The figure shows three views and two pictorial views of one solid part (mm, origin at its lowest corner). Answer the questions. A direction names the side the tool comes from. Coordinates: 2 decimals unless noted, no trailing zeros. Loops run counter-clockwise (first coordinate to the right, second up) from the corner with the lowest first, then second, coordinate; pieces in that order, holes last. Notation, with made-up numbers: M 38.5,-23 L 87.5,-23 A14 ccw 87.5,-6 Z; hole C 65.25,-21 d2. An arc over 180 degrees is marked long. Return JSON: item names as keys, results as strings. Group by question number.
1. Given P1, Ø3, axis at x = 20.5, z = 108.5, coming from the -Y side; P2, Ø2, axis at y = 323.5, z = 159.5, coming from the -X side; P3, Ø3, axis at x = 5.5, y = 253.5, coming from the +Z side; P4, Ø6, axis at x = 21, z = 110, coming from the +Y side, each flat-ended and moving along its own axis, determine where each tip first touches the part or whether it passes through.
2. The mould has two halves that part along Y. Classify the marked faces 1, 2, 3 and 4: pulls with the +Y half, pulls with the -Y half, needs draft (parallel to the pull), parting line crosses it, or undercut.
3. Straight lines are drawn through the part: L1, parallel to Z at x = 8.5, y = 28.5; L2, parallel to Z at x = 1.5, y = 92.5; L3, parallel to Y at x = 19.75, z = 166. For each, find the intervals that lie inside material, in ascending order. Write a range as from..to.
4. Section C-C (y = 89.5) is taken. Write down the section's boundary in (x, z), then the cut area to 3 significant figures.
5. Which of the six approach directions +Z, -Z, +X, -X, +Y, -Y give full straight-line access (tool end or side, diameter ignored) to the marked faces 5, 6 and 7?
6. Section B-B (z = 73.5) is taken. Write down the section's boundary in (x, y).
7. Section A-A (x = 18.75) is taken. Write down the section's boundary in (y, z), then the cut area to 3 significant figures.
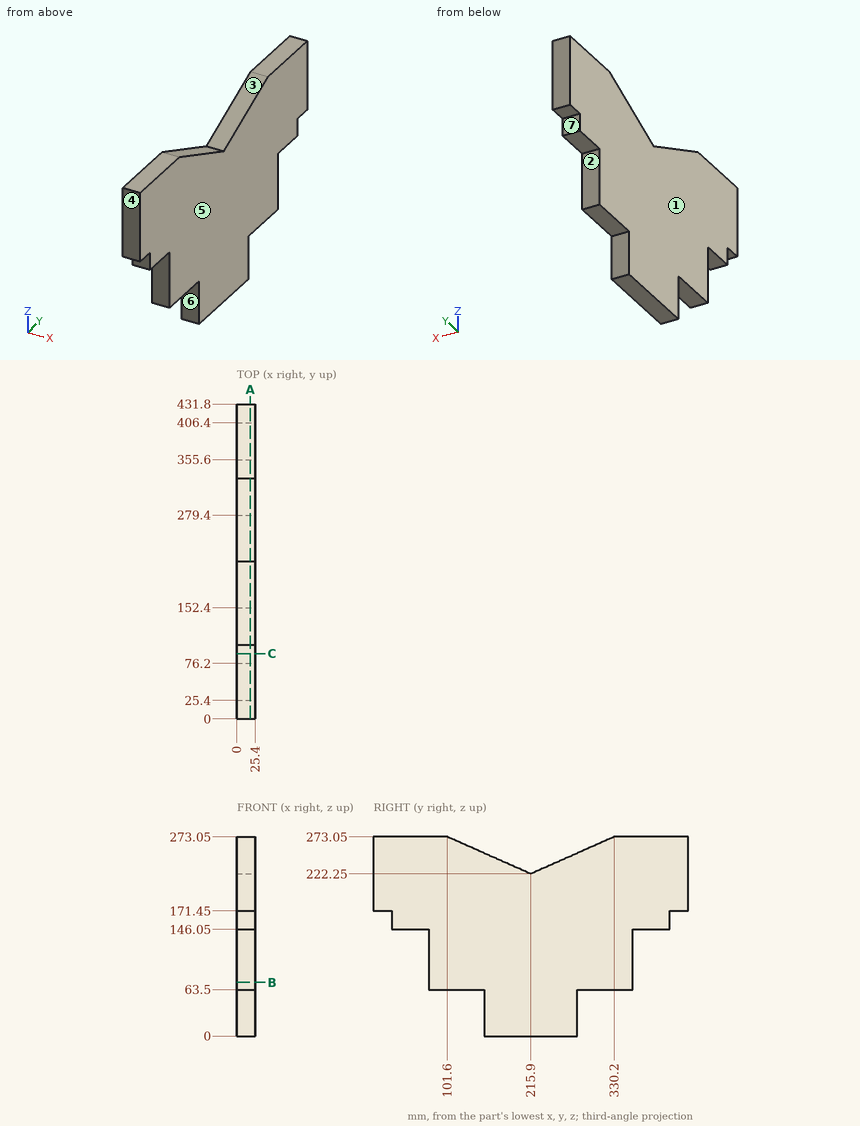
Worked out:
{
 "1": {"P1": "y = 76.2", "P2": "x = 0", "P3": "z = 239.63", "P4": "y = 355.6"},
 "2": {"face 1": "needs draft", "face 2": "pulls with the +Y half", "face 3": "undercut", "face 4": "pulls with the -Y half"},
 "3": {"L1": "146.05..273.05", "L2": "63.5..273.05", "L3": "25.4..406.4"},
 "4": {"outline": "M 0,63.5 L 25.4,63.5 L 25.4,273.05 L 0,273.05 Z", "area": "5,320 mm^2"},
 "5": {"face 5": "+Z, -Z, +X, +Y, -Y", "face 6": "-Z, +X, -X, -Y", "face 7": "-Z, +X, -X, +Y"},
 "6": {"outline": "M 0,76.2 L 25.4,76.2 L 25.4,355.6 L 0,355.6 Z"},
 "7": {"outline": "M 0,171.45 L 25.4,171.45 L 25.4,146.05 L 76.2,146.05 L 76.2,63.5 L 152.4,63.5 L 152.4,0 L 279.4,0 L 279.4,63.5 L 355.6,63.5 L 355.6,146.05 L 406.4,146.05 L 406.4,171.45 L 431.8,171.45 L 431.8,273.05 L 330.2,273.05 L 215.9,222.25 L 101.6,273.05 L 0,273.05 Z", "area": "78,900 mm^2"}
}
